For this review, use the dimensioned drawing (mm, ordinates from the lowest corner) and the shaded views. Give positions to 0.01 mm unless a question says otherwise; leave off trailing zeros. Write each loop counter-clockwise with the first axis right and the second up, starting at its lowest first coordinate (ties: lowest second). Pieces come first, ordered by that corner, then holes. Notation, with made-up numbers: M -4,35.5 L 54,35.5 A21 ccw 54,59.5 Z; hole C 60.25,29.5 d1. An arc over 180 degrees is marked long. Answer in a Markdown table with one row per item.
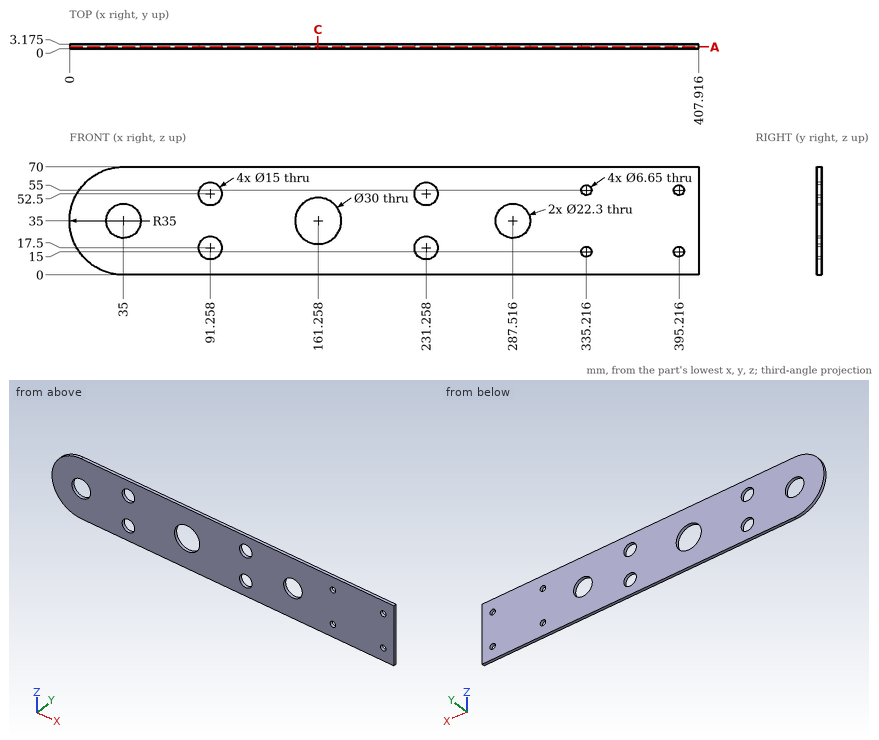
1) To check wall thickness, follow probe 1 along Z at (x, y) = (162, 1.55); probe 2 along X at (y, z) = (2, 51) (1 decimal); probe 3 along X at (y, z) = (2.15, 36) (1 decimal). State the ranges of each line that lie inside material, in increasing order. Write a range as [from, to].
Geometry says:
| item | result |
|---|---|
| probe 1 | [0, 20.02], [49.98, 70] |
| probe 2 | [3.9, 83.9], [98.6, 223.9], [238.6, 407.9] |
| probe 3 | [0, 23.9], [46.1, 146.3], [176.2, 276.4], [298.6, 407.9] |
2) Add section A-A (y = 1.3). Count the separate pieces of the cut face and the enclosed holes in it, and give its area (3 significant figures).
Geometry says:
| item | result |
|---|---|
| separate pieces | 1 |
| enclosed holes | 11 |
| area | 25,700 mm^2 |
3) Add section C-C (x = 161). Write out the cut boundary in (y, z) (1 decimal), and give its area (3 significant figures).
Geometry says:
| item | result |
|---|---|
| outline | M 0,0 L 3.2,0 L 3.2,20 L 0,20 Z; M 0,50 L 3.2,50 L 3.2,70 L 0,70 Z |
| area | 127 mm^2 |
